Print and shaded views of the part. All mm, measured from the part's lowest x, y and z. A direction names the side the tool comes from. Round coordinates to 2 decimals unless told otherwise and drop trailing zeros. Order: outer loops, then holes, each group sorted by start corner. A loop starts at its lowest first (then second) coordinate and runs counter-clockwise, first axis right, second up. Notation, with made-up numbers: (45.25, 0.5) - (60.25, 0.5) arc R30 cw to (60.25, 36.5) - close; hole circle Ø11 at (43.25, 23). An arc over 180 degrees is marked (long way). Write item = value, one per line.
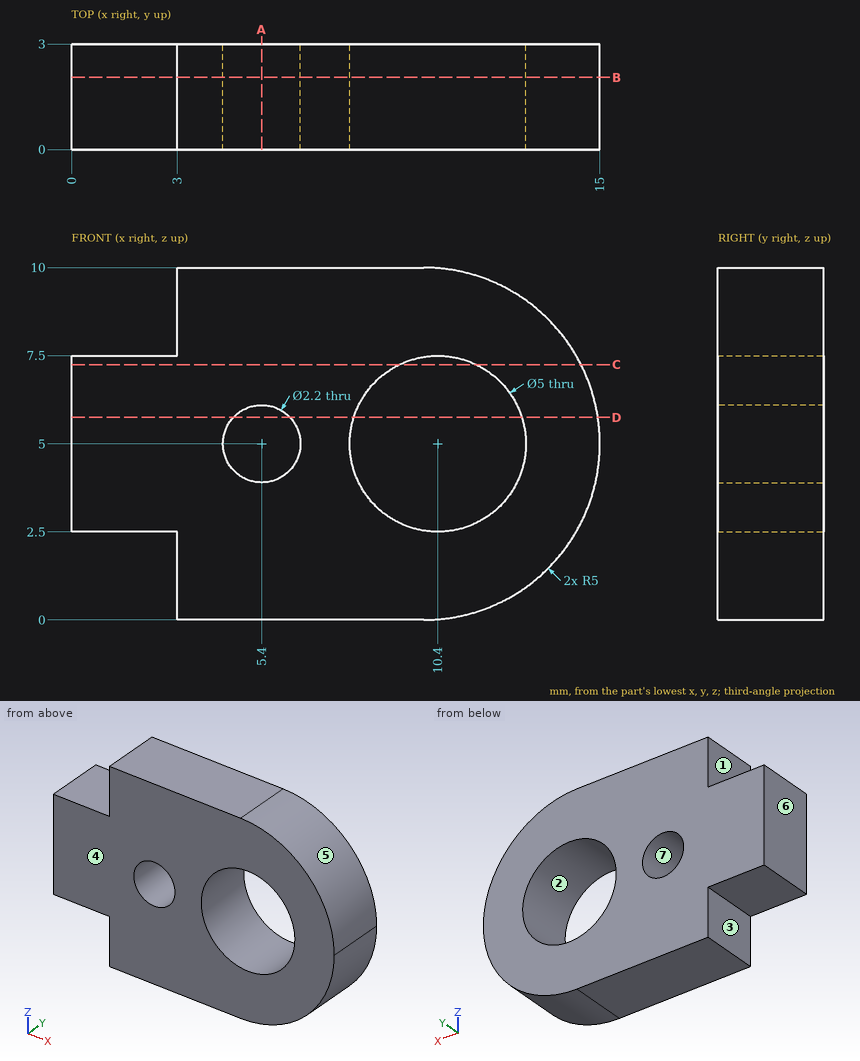
(1) Pull direction X, two halves, no side cores. Call the marked faces 4, 5, 6 and 7: released by +X, released by -X, zero draft, split by the parting line, or undercut.
Solved:
face_4 = zero draft
face_5 = released by +X
face_6 = released by -X
face_7 = undercut
(2) Band-saw the part on B-B on y = 2.05. Count the separate pieces of the cut face and the enclosed holes in it, plus the area to 3 significant figures.
Solved:
separate_pieces = 1
enclosed_holes = 2
area = 101 mm²
(3) Band-saw the part on A-A on x = 5.4. List the corners of the cut face in (y, z).
Solved:
outline = (0, 0) - (3, 0) - (3, 3.9) - (0, 3.9) - close; (0, 6.1) - (3, 6.1) - (3, 10) - (0, 10) - close
(4) Probe line 1 along X through (y, z) = (2.25, 5); line 2 along X through (y, z) = (1.2, 4.5) (1 decimal); line 3 along Z through (x, y) = (4.5, 2.05). List the from-to ranges inside material, lowest first.
Solved:
line_1 = 0 to 4.3, 6.5 to 7.9, 12.9 to 15
line_2 = 0 to 4.4, 6.4 to 8, 12.8 to 15
line_3 = 0 to 4.37, 5.63 to 10
(5) Band-saw the part on D-D on z = 5.75. List the corners of the cut face in (x, y) (1 decimal), plus the area to 3 significant figures.
Solved:
outline = (0, 0) - (4.6, 0) - (4.6, 3) - (0, 3) - close; (6.2, 0) - (8, 0) - (8, 3) - (6.2, 3) - close; (12.8, 0) - (14.9, 0) - (14.9, 3) - (12.8, 3) - close
area = 25.7 mm²
(6) Tool access for the marked faces 1, 2 and 3: list every direction of +Z, -Z, +X, -X, +Y, -Y with a clear straight run to the whole face (end or side of a thin tool).
Solved:
face_1 = +Z, -X, +Y, -Y
face_2 = +Y, -Y
face_3 = -Z, -X, +Y, -Y
(7) Band-saw the part on C-C on z = 7.25. List the corners of the cut face in (x, y) (3 decimals).
Solved:
outline = (0, 0) - (9.31, 0) - (9.31, 3) - (0, 3) - close; (11.49, 0) - (14.465, 0) - (14.465, 3) - (11.49, 3) - close
(8) Drop flat-ended pins along their axis: pin 1 (1 mm diameter, centred on y = 1, z = 7, fed in from -X); pin 2 (1.2 mm diameter, centred on y = 2, z = 1.5, fed in from -X); pin 3 (0.9 mm diameter, centred on x = 1.5, y = 1, fed in from +Z). Give the stop position or say it passes through.
Solved:
pin_1 = 0
pin_2 = 3
pin_3 = 7.5
